The listing builds one solid part. Answer for the finished solid, in the listing's coordinates (mm). Round coordinates to 2 decimals unless told otherwise and drop trailing zeros. Write each loop counter-clockwise with the first axis right and the second up, starting at its lowest first coordinate (ties: lowest second). Pieces come first, ordered by that corner, then holes. Notation, with made-up numbers: (31, 8.5) - (39, 8.5) arc R8 cw to (39, 16.5) - close; hole circle Ø3 at (-10.75, 30.5). An arc over 180 degrees is marked (long way). Answer in a Markdown table with one row per item.
from build123d import *

# Parameters (mm, degrees)
SKETCH_1_R          = 2.1
EXTRUDE_1_DEPTH     = 5.6
SKETCH_2_W          = 20
SKETCH_2_H          = 15.8
SKETCH_2_R          = 1.6
EXTRUDE_2_DEPTH     = 5.6
SKETCH_3_R          = 1.6
CUT_EXTRUDE_1_DEPTH = 199.148738326
SKETCH_4_W          = 50
SKETCH_4_H          = 53.03030303
SKETCH_4_W_2        = 120
SKETCH_4_H_2        = 20
CUT_EXTRUDE_2_DEPTH = 199.148738326
SKETCH_6_W          = 90
SKETCH_6_H          = 10
CUT_EXTRUDE_3_DEPTH = 199.148738326
SKETCH_7_W          = 30
SKETCH_7_H          = 10
EXTRUDE_3_DEPTH     = 5.6
FILLET_1_R          = 3
FILLET_2_R          = 5
FILLET_3_R          = 2


with BuildPart() as part:
    # ｽｹｯﾁ1 → ﾎﾞｽ - 押し出し1 (new body)
    with BuildSketch(Plane(origin=(0, 0, 0), x_dir=(1, 0, 0), z_dir=(0, 1, 0))):
        Polygon((-147, 36.75), (-147, -36.75), (147, -36.75), (147, 36.75), (75, 132.75), (-75, 132.75), align=None)
        with Locations(Location((140, 37.75, 0), (0, 0, 270))):
            Circle(SKETCH_1_R, mode=Mode.SUBTRACT)
        with Locations(Location((-140, 37.75, 0), (0, 0, 270))):
            Circle(SKETCH_1_R, mode=Mode.SUBTRACT)
        with Locations(Location((125, 57.75, 0), (0, 0, 270))):
            Circle(SKETCH_1_R, mode=Mode.SUBTRACT)
        with Locations(Location((-125, 57.75, 0), (0, 0, 270))):
            Circle(SKETCH_1_R, mode=Mode.SUBTRACT)
    extrude(amount=EXTRUDE_1_DEPTH)

    # ｽｹｯﾁ2 → ﾎﾞｽ - 押し出し2 (add)
    # profile 1 of 2: a face of its own
    with BuildSketch(Plane(origin=(0, 0, 0), x_dir=(1, 0, 0), z_dir=(0, 1, 0))):
        with Locations((-85, -44.65)):
            Rectangle(SKETCH_2_W, SKETCH_2_H)
        with Locations(Location((-85, -47.55, 0), (0, 0, 270))):
            Circle(SKETCH_2_R, mode=Mode.SUBTRACT)
    # profile 2 of 2: a face of its own
    with BuildSketch(Plane(origin=(0, 0, 0), x_dir=(1, 0, 0), z_dir=(0, 1, 0))):
        with Locations((85, -44.65)):
            Rectangle(SKETCH_2_W, SKETCH_2_H)
        with Locations(Location((85, -47.55, 0), (0, 0, 90))):
            Circle(SKETCH_2_R, mode=Mode.SUBTRACT)
    extrude(amount=EXTRUDE_2_DEPTH)

    # ｽｹｯﾁ3 → ｶｯﾄ - 押し出し1 (cut, through all)
    with BuildSketch(Plane(origin=(0, 5.6, 0), x_dir=(1, 0, 0), z_dir=(0, 1, 0))):
        with Locations(Location((36, 77.75, 0), (0, 0, 270))):
            Circle(SKETCH_3_R)
        with Locations(Location((-30, 77.75, 0), (0, 0, 90))):
            Circle(SKETCH_3_R)
        with Locations(Location((-30, 7.75, 0), (0, 0, 270))):
            Circle(SKETCH_3_R)
        with Locations(Location((36, 7.75, 0), (0, 0, 90))):
            Circle(SKETCH_3_R)
        with Locations(Location((-92.005, 48.19, 0), (0, 0, 270))):
            Circle(SKETCH_3_R)
        with Locations(Location((-92.005, -2.69, 0), (0, 0, 90))):
            Circle(SKETCH_3_R)
        with Locations(Location((-121.995, -2.69, 0), (0, 0, 270))):
            Circle(SKETCH_3_R)
        with Locations(Location((-121.995, 48.19, 0), (0, 0, 90))):
            Circle(SKETCH_3_R)
    extrude(amount=-CUT_EXTRUDE_1_DEPTH, mode=Mode.SUBTRACT)

    # ｽｹｯﾁ4 → ｶｯﾄ - 押し出し2 (cut, through all)
    with BuildSketch(Plane(origin=(0, 5.6, 0), x_dir=(1, 0, 0), z_dir=(0, 1, 0))):
        Polygon((-87.5, 82.75), (87.5, 82.75), (65, 112.75), (-65, 112.75), align=None)
        with Locations((3, 42.75)):
            Rectangle(SKETCH_4_W, SKETCH_4_H)
        with Locations((0, -16.75)):
            Rectangle(SKETCH_4_W_2, SKETCH_4_H_2)
    extrude(amount=-CUT_EXTRUDE_2_DEPTH, mode=Mode.SUBTRACT)

    # ｽｹｯﾁ6 → ｶｯﾄ - 押し出し3 (cut, through all)
    with BuildSketch(Plane(origin=(0, 5.6, 0), x_dir=(1, 0, 0), z_dir=(0, 1, 0))):
        with Locations((0, 127.75)):
            Rectangle(SKETCH_6_W, SKETCH_6_H)
    extrude(amount=-CUT_EXTRUDE_3_DEPTH, mode=Mode.SUBTRACT)

    # ｽｹｯﾁ7 → ﾎﾞｽ - 押し出し3 (add)
    with BuildSketch(Plane(origin=(0, 5.6, 0), x_dir=(1, 0, 0), z_dir=(0, 1, 0))):
        with Locations((0, 127.75)):
            Rectangle(SKETCH_7_W, SKETCH_7_H)
    extrude(amount=-EXTRUDE_3_DEPTH)

    # ﾌｨﾚｯﾄ1
    fillet_1_edges = [part.edges().sort_by_distance(p)[0] for p in [
        (-87.5, 2.8, -82.75),
        (-65, 2.8, -112.75),
        (65, 2.8, -112.75),
        (87.5, 2.8, -82.75),
        (28, 2.8, -69.265151515),
        (28, 2.8, -16.234848485),
        (-22, 2.8, -16.234848485),
        (-22, 2.8, -69.265151515),
        (60, 2.8, 26.75),
        (-60, 2.8, 26.75),
        (-60, 2.8, 6.75),
        (60, 2.8, 6.75),
    ]]
    fillet(fillet_1_edges, radius=FILLET_1_R)

    # ﾌｨﾚｯﾄ2
    fillet_2_edges = [part.edges().sort_by_distance(p)[0] for p in [
        (-147, 2.8, 36.75),
        (-147, 2.8, -36.75),
        (-75, 2.8, -132.75),
        (75, 2.8, -132.75),
        (147, 2.8, -36.75),
        (147, 2.8, 36.75),
        (45, 2.8, -132.75),
        (45, 2.8, -122.75),
        (-45, 2.8, -132.75),
        (-45, 2.8, -122.75),
        (15, 2.8, -132.75),
        (15, 2.8, -122.75),
        (-15, 2.8, -132.75),
        (-15, 2.8, -122.75),
    ]]
    fillet(fillet_2_edges, radius=FILLET_2_R - 0.0001)  # a hair under: the kernel refuses the full size

    # ﾌｨﾚｯﾄ3
    fillet_3_edges = [part.edges().sort_by_distance(p)[0] for p in [
        (-95, 2.8, 52.55),
        (-75, 2.8, 52.55),
        (75, 2.8, 52.55),
        (95, 2.8, 52.55),
    ]]
    fillet(fillet_3_edges, radius=FILLET_3_R)


solid = part.part
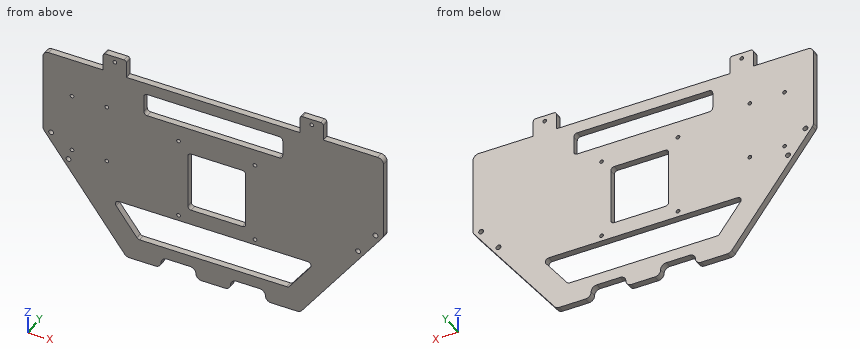
(1) Section B-B (z = -108.5) is taken. Give the vertices of the cut face in (x, y), and give its area (3 significant figures).
Checked values:
| item | result |
|---|---|
| outline | (-93.19, 0) - (-68.19, 0) - (-68.19, 5.6) - (-93.19, 5.6) - close; (68.19, 0) - (93.19, 0) - (93.19, 5.6) - (68.19, 5.6) - close |
| area | 280 mm2 |
(2) Section A-A (x = -69.5) is taken. Give the vertices of the cut face in (y, z), and give its area (3 significant figures).
Checked values:
| item | result |
|---|---|
| outline | (0, -132.75) - (5.6, -132.75) - (5.6, -106.75) - (0, -106.75) - close; (0, -82.75) - (5.6, -82.75) - (5.6, 36.75) - (0, 36.75) - close |
| area | 815 mm2 |
(3) Find the intervals of material crossed by line 1 (Z direction, x = 52.5, y = 1.2); line 2 (X direction, y = 3.3, z = 2.69) (3 decimals); line 3 (Z direction, x = -36.5, y = 1.1), in increasing order.
Checked values:
| item | result |
|---|---|
| line 1 | z = -132.75 to -112.75, -82.75 to 6.75, 26.75 to 36.75 |
| line 2 | x = -147 to -123.595, -120.395 to -93.605, -90.405 to 147 |
| line 3 | z = -122.75 to -112.75, -82.75 to 6.75, 26.75 to 36.75 |
(4) Flat-ended cylindrical pins translate along their axes: pin 1 (1.5 mm diameter, centred on x = -112, y = 3.5, fed in from -Z); pin 2 (2 mm diameter, centred on x = 116, y = 4, fed in from -Z); pin 3 (1.7 mm diameter, centred on x = 29, y = 4, fed in from +Z). Find the tip coordinate at first contact, or state that the pin passes through.
Checked values:
| item | result |
|---|---|
| pin 1 | stops at z = -84.42 |
| pin 2 | stops at z = -79.42 |
| pin 3 | stops at z = 36.75 |
(5) Section C-C (y = 4.5) is taken. State how many separate pieces and enclosed holes the cut face has, and give its area (3 significant figures).
Checked values:
| item | result |
|---|---|
| separate pieces | 1 |
| enclosed holes | 17 |
| area | 33,200 mm2 |
